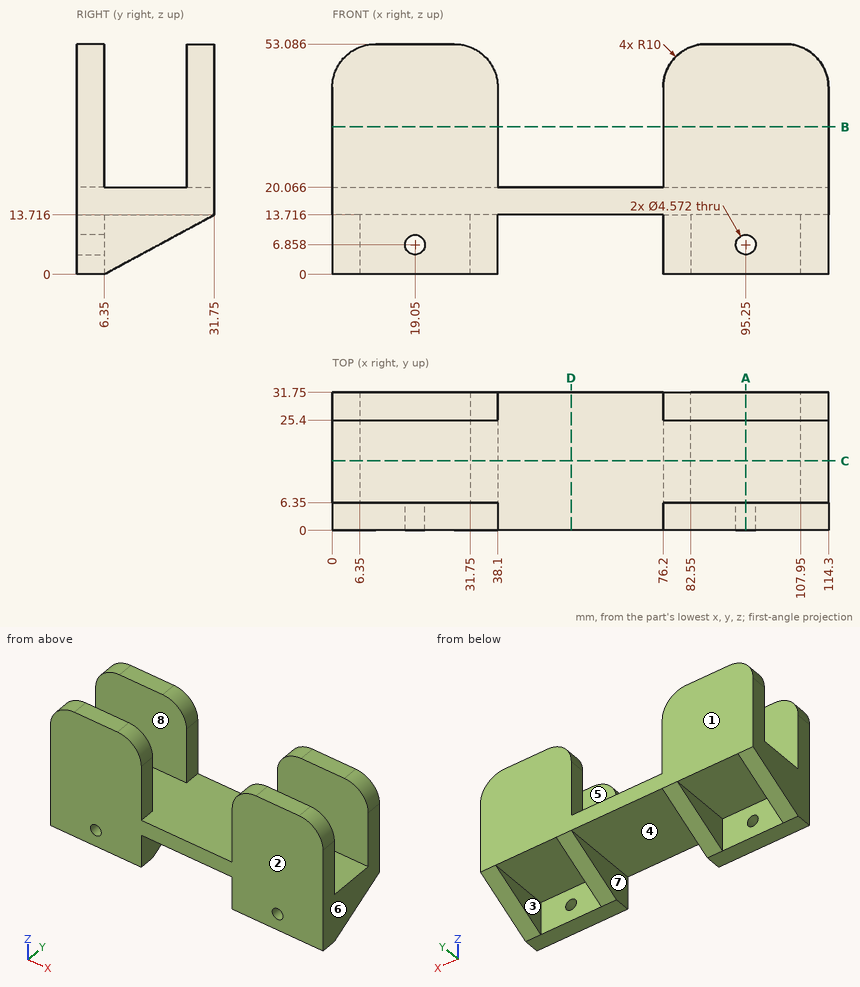
Check sheet for the drawn part. Datum: minimum x, y, z corner. Units: mm. A direction names the side the tool comes from. Round coordinates to 2 decimals unless told otherwise and drop trailing zeros. Order: outer loops, then holes, each group sorted by start corner. A loop starts at its lowest first (then second) coordinate and runs counter-clockwise, first axis right, second up.
(1) Access from +Z, -Z, +X, -X, +Y, -Y to the whole of each face (thin tool, end or side, straight path). Record for the marked faces 1, 2, 3, 4 and 5.
(2) Cross-section at D-D, the plane x = 55. Enter the section's corners in (y, z).
(3) Cross-section at A-A, the plane x = 95.25. Enter the section's corners in (y, z).
(4) Go/stop test with flat-tipped pins: P1, Ø4, axis at x = 64, y = 17.5, coming from the -Z side; P2, Ø6, axis at x = 42.5, y = 3.5, coming from the +Z side. Record where each tip stops, or that it passes through.
(5) Draft check along X on the marked faces 6, 7 and 8. Enter one of: pulls with the +X half, pulls with the -X half, needs draft (parallel to the pull), parting line crosses it, or undercut.
(6) Cross-section at B-B, the plane z = 34. Enter the section's corners in (x, y), and give its area (3 significant figures).
(7) Scan lines: probe 1 along X at (y, z) = (22, 11.5); probe 2 along Y at (x, z) = (89, 23.5); probe 3 along X at (y, z) = (4, 26.5). Record each from-to range of solid material in increasing order.
(8) Cross-section at C-C, the plane y = 16. Enter the section's corners in (x, z).
Check sheet entries:
1. face 1: +Z, -Z, +X, -X, +Y
1. face 2: +Z, -Z, +X, -X, -Y
1. face 3: -Z, +Y
1. face 4: -Z, +Y, -Y
1. face 5: +Z, +X, -X
2. outline: (0, 13.72) - (31.75, 13.72) - (31.75, 20.07) - (0, 20.07) - close
3. outline: (0, 0) - (6.35, 0) - (6.35, 4.57) - (0, 4.57) - close; (0, 9.14) - (6.35, 9.14) - (6.35, 13.72) - (31.75, 13.72) - (31.75, 53.09) - (25.4, 53.09) - (25.4, 20.07) - (6.35, 20.07) - (6.35, 53.09) - (0, 53.09) - close
4. P1: stops at z = 13.72
4. P2: stops at z = 20.07
5. face 6: pulls with the +X half
5. face 7: undercut
5. face 8: needs draft
6. outline: (0, 0) - (38.1, 0) - (38.1, 6.35) - (0, 6.35) - close; (0, 25.4) - (38.1, 25.4) - (38.1, 31.75) - (0, 31.75) - close; (76.2, 0) - (114.3, 0) - (114.3, 6.35) - (76.2, 6.35) - close; (76.2, 25.4) - (114.3, 25.4) - (114.3, 31.75) - (76.2, 31.75) - close
6. area: 968 mm2
7. probe 1: x = 0 to 6.35, 31.75 to 38.1, 76.2 to 82.55, 107.95 to 114.3
7. probe 2: y = 0 to 6.35, 25.4 to 31.75
7. probe 3: x = 0 to 38.1, 76.2 to 114.3
8. outline: (0, 5.21) - (6.35, 5.21) - (6.35, 13.72) - (31.75, 13.72) - (31.75, 5.21) - (38.1, 5.21) - (38.1, 13.72) - (76.2, 13.72) - (76.2, 5.21) - (82.55, 5.21) - (82.55, 13.72) - (107.95, 13.72) - (107.95, 5.21) - (114.3, 5.21) - (114.3, 20.07) - (0, 20.07) - close
